Autodesk Fusion 360 part; units mm, degrees
cylinder "CylinderPrimitive1" add diameter 28 height 71 placed x (1, 0, 0) y (0, 0, -1) z (0, 1, 0) at (0, 0, 0) makes body 1
cylinder "CylinderPrimitive2" add diameter 22 height 82 placed x (1, 0, 0) y (0, 0, -1) z (0, 1, 0) at (0, 0, 0) bodies 1
hole "Hole1" at (0, 82, 0) direction (0, -1, 0) diameter 18 end through all bodies 1 1
cylinder "CylinderPrimitive3" add diameter 28 height 35 placed x (1, 0, 0) y (0, 1, 0) z (0, 0, 1) at (0, 0, 0) bodies 1
box "BoxPrimitive1" add length 16 width 90 height 32 placed x (0, 1, 0) y (0, 0, 1) z (1, 0, 0) at (0, -16, -11) separate body makes body 2
move_body "Move1" bodies 2 to x (1, 0, 0) y (0, 1, 0) z (0, 0, 1) at (-16, 0, 0)
sphere "SpherePrimitive1" add diameter 28 placed x (1, 0, 0) y (0, 1, 0) z (0, 0, 1) at (0, 0, 35) bodies 1
combine "Combine1" operation cut target body 1 tool bodies 2
hole "Hole2" at (0, 0, 0) direction (0, 1, 0) diameter 19 depth 15 tip angle 118 bodies 1
hole "Hole3" at (0.1519, 0, 30.6055) direction (0, 1, 0) diameter 1.623 depth 6 tip angle 118 counterbore diameter 2 counterbore depth 1 bodies 1
CAD build for the part. Positions are in the model's coordinates, mm. A direction names the side the tool comes from. Give positions to 0.01 mm unless a question says otherwise; leave off trailing zeros. Order: outer loops, then holes, each group sorted by start corner. A loop starts at its lowest first (then second) coordinate and runs counter-clockwise, first axis right, second up.
(1) Tool access for faces 1 (the cylindrical face through (8.43, 7.6, -4.38)), 2 (the cylindrical face through (-8.923, 48.183, -1.172)), 3 (the flat face through (2, 82, 9)), 4 (the cylindrical face through (-2.38, 76.58, 10.74)), 5 (the cylindrical face through (0, 14, 22)): list every direction of +Z, -Z, +X, -X, +Y, -Y with a clear straight run to the whole face (end or side of a thin tool).
(2) Drill centre lines: L1, parallel to X at y = 6, z = 0; L2, parallel to X at y = 64, z = 0; L3, parallel to Y at x = 2.75, z = 11. Where is each one in solid material? Low to high.
(3) Flat gauge pins, fed straight in: pin 1 (5 mm diameter, centred on x = 8, y = 18, fed in from +Z); pin 2 (2.5 mm diameter, centred on x = 0.15, z = 30.61, fed in from -Y); pin 3 (4 mm diameter, centred on y = 13.5, z = 25.5, fed in from -X); pin 4 (1 mm diameter, centred on x = 0, z = 30.5, fed in from -Y). Where does each tip first touch, or does it go through?
(4) Mould opens along X. For faces 6 (the flat face through (6.2, 71, 9.3)), 7 (the cylindrical face through (-1.82, 36, -13.88)), 8 (the cylindrical face through (0.108, 0.507, 31.605)) say: released by +X, released by -X, zero draft, split by the parting line, or undercut.
(5) Saw through at A-A, the plane y = 17. Give the cut face in (x, z).
(6) Saw through at B-B, the plane z = 40.5. Give the cut face in (x, y).
(7) Saw through at C-C, the plane y = 72. Give the cut face in (x, z).
Results found:
1. face 1: -Y
1. face 2: +Y, -Y
1. face 3: +Z, -Z, +X, -X, +Y
1. face 4: +Y
1. face 5: +Z, +Y
2. L1: x = -14 to -9.5, 9.5 to 14
2. L2: x = -14 to -9, 9 to 14
2. L3: y = 0 to 71
3. pin 1: stops at z = 12.87
3. pin 2: stops at y = 0
3. pin 3: stops at x = -7.98
3. pin 4: stops at y = 6.08
4. face 6: zero draft
4. face 7: split by the parting line
4. face 8: undercut
5. outline: circle Ø28 at (0, 0); hole circle Ø18 at (0, 0)
6. outline: (-12.87, 0) - (12.87, 0) arc R12.87 ccw to start
7. outline: circle Ø22 at (0, 0); hole circle Ø18 at (0, 0)
